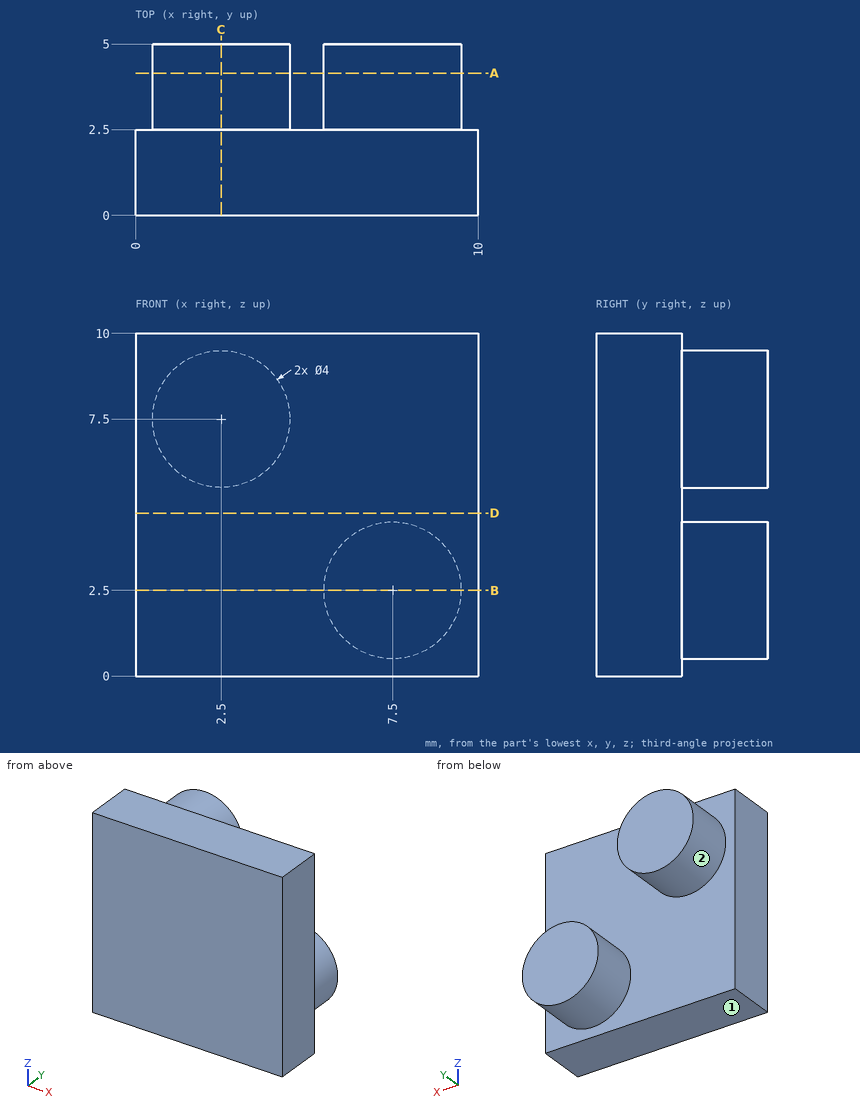
Could you check a few things on this drawing? It's one solid part, dimensions in mm from its lowest x, y, z. A direction names the side the tool comes from. Round coordinates to 2 decimals unless told otherwise and drop trailing zeros. Loops run counter-clockwise (first coordinate to the right, second up) from the corner with the lowest first, then second, coordinate; pieces in that order, holes last.
Q1. On a 3-axis mill with a long thin cutter (end or side, diameter ignored), from which of +Z, -Z, +X, -X, +Y, -Y can I reach the whole of each face in a straight line? I mean the marked faces 1 and 2. Say none if no direction works.
Q2. I want a section at B-B (z = 2.5). Write out the boundary of the cut face in (x, y), and give its area (3 significant figures).
Q3. Please list where these lines run through material, in increasing order: L1, parallel to Y at x = 7.25, z = 9; L2, parallel to Z at x = 1, y = 3.8; L3, parallel to X at y = 4.75, z = 8.5.
Q4. I want a section at C-C (x = 2.5). Write out the boundary of the cut face in (y, z), and give its area (3 significant figures).
Q5. For P1, Ø3, axis at x = 7, z = 8, coming from the +Y side; P2, Ø1.5, axis at y = 3.5, z = 2, coming from the -X side, each with a flat end and sliding along its axis, tell me the tip position at first contact or that it passes through.
Q6. I want a section at D-D (z = 4.75). Write out the boundary of the cut face in (x, y), and give its area (3 significant figures).
Q7. I want a section at A-A (y = 4.15). Write out the boundary of the cut face in (x, z), and give its area (3 significant figures).
Answer below:
1. face 1: -Z, +X, -X, +Y, -Y
1. face 2: +Y
2. outline: (0, 0) - (10, 0) - (10, 2.5) - (9.5, 2.5) - (9.5, 5) - (5.5, 5) - (5.5, 2.5) - (0, 2.5) - close
2. area: 35.0 mm2
3. L1: y = 0 to 2.5
3. L2: z = 6.18 to 8.82
3. L3: x = 0.77 to 4.23
4. outline: (0, 0) - (2.5, 0) - (2.5, 5.5) - (5, 5.5) - (5, 9.5) - (2.5, 9.5) - (2.5, 10) - (0, 10) - close
4. area: 35.0 mm2
5. P1: stops at y = 2.5
5. P2: stops at x = 5.5
6. outline: (0, 0) - (10, 0) - (10, 2.5) - (0, 2.5) - close
6. area: 25.0 mm2
7. outline: circle Ø4 at (2.5, 7.5); circle Ø4 at (7.5, 2.5)
7. area: 25.1 mm2
